Part print with two shaded views. Sizes in mm from the minimum x, y, z corner. A direction names the side the tool comes from. Round coordinates to 2 decimals unless told otherwise and drop trailing zeros. Write each loop counter-clockwise with the first axis right and the second up, starting at its lowest first coordinate (ties: lowest second). Pieces come first, ordered by that corner, then holes. Notation, with made-up numbers: (-24.75, -12) -> (-9.75, -12) arc R8 cw to (-9.75, 0) -> close; hole circle Ø8 at (-29, -36). An arc over 180 degrees is marked (long way). Return JSON: item names as keys, results as strings.
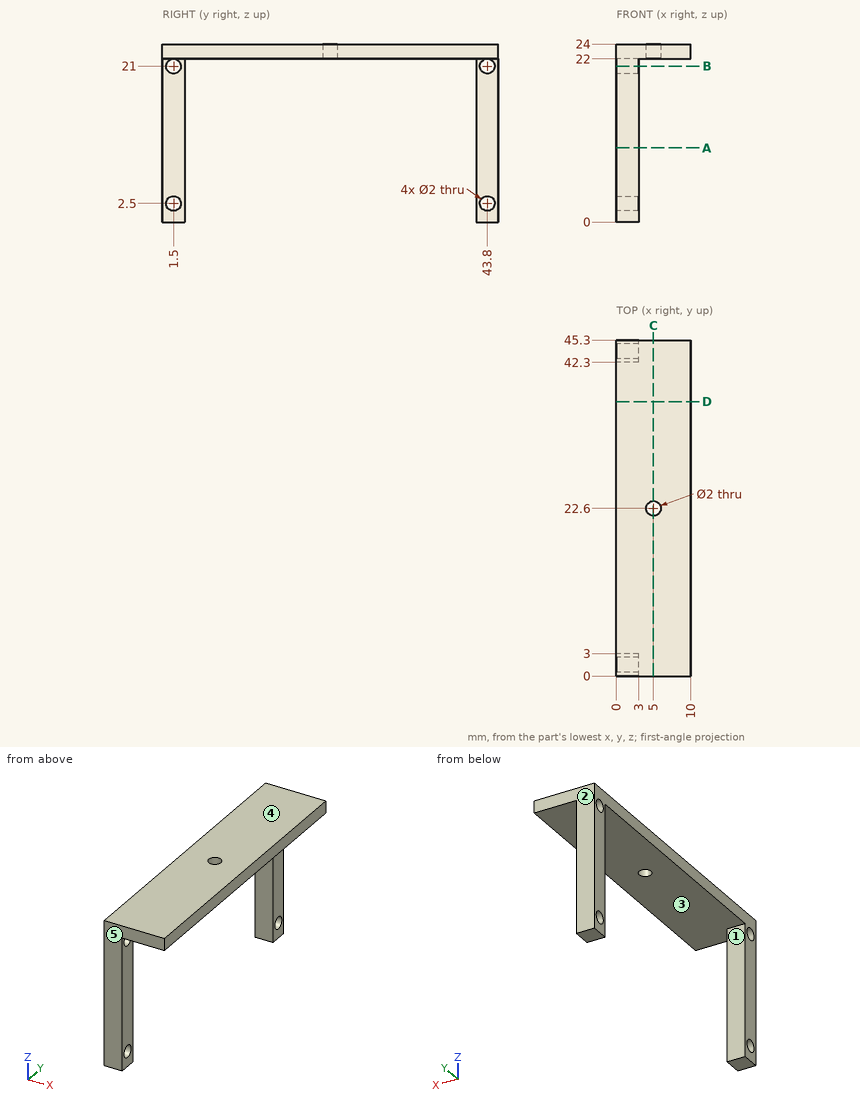
Q1. Saw through at B-B on z = 21. List the corners of the cut face in (x, y), then the cut area to 3 significant figures.
Verdict:
{"outline": "(0, 0) -> (3, 0) -> (3, 0.5) -> (0, 0.5) -> close; (0, 2.5) -> (3, 2.5) -> (3, 3) -> (0, 3) -> close; (0, 42.3) -> (3, 42.3) -> (3, 42.8) -> (0, 42.8) -> close; (0, 44.8) -> (3, 44.8) -> (3, 45.3) -> (0, 45.3) -> close", "area": "6.00 mm²"}
Q2. Wall check: L1, parallel to Z at x = 1.9, y = 43.8; L2, parallel to Y at x = 1, z = 2.5; L3, parallel to Z at x = 2.5, y = 7. Give the ranges that are in metal, low to high.
Verdict:
{"L1": "z = 0 to 1.5, 3.5 to 20, 22 to 24", "L2": "y = 0 to 0.5, 2.5 to 3, 42.3 to 42.8, 44.8 to 45.3", "L3": "z = 22 to 24"}
Q3. 3-axis set-ups, long thin cutter, end or side, ignore diameter. For the marked faces 1 and 2: which of +Z, -Z, +X, -X, +Y, -Y reach the whole face in a straight line?
Verdict:
{"face 1": "-Z, +X, -X", "face 2": "+Z, -Z, +X, -X, +Y"}
Q4. Two-plate mould, pull along Y, no slides. Class the marked faces 3, 4 and 5: +Y half, -Y half, draft (parallel to the pull), parting line (faces both ways), or undercut.
Verdict:
{"face 3": "undercut", "face 4": "draft", "face 5": "-Y half"}
Q5. Saw through at C-C on x = 5. List the corners of the cut face in (y, z).
Verdict:
{"outline": "(0, 22) -> (21.6, 22) -> (21.6, 24) -> (0, 24) -> close; (23.6, 22) -> (45.3, 22) -> (45.3, 24) -> (23.6, 24) -> close"}
Q6. Saw through at A-A on z = 10. List the corners of the cut face in (x, y), then the cut area to 3 significant figures.
Verdict:
{"outline": "(0, 0) -> (3, 0) -> (3, 3) -> (0, 3) -> close; (0, 42.3) -> (3, 42.3) -> (3, 45.3) -> (0, 45.3) -> close", "area": "18.0 mm²"}
Q7. Pin check, flat tips, straight feed: pin 1 Ø1.8 at (y, z) = (1.5, 21) entering from -X; pin 2 Ø0.9 at (y, z) = (43.5, 11.5) entering from +X; pin 3 Ø3 at (x, y) = (5, 17.5) entering from -Z. Stop position of each tip, or through.
Verdict:
{"pin 1": "passes through", "pin 2": "stops at x = 3", "pin 3": "stops at z = 22"}
Q8. Saw through at D-D on y = 37. List the corners of the cut face in (x, z), then the cut area to 3 significant figures.
Verdict:
{"outline": "(0, 22) -> (10, 22) -> (10, 24) -> (0, 24) -> close", "area": "20.0 mm²"}
